Part model, mm, in its own coordinate system. A direction names the side the tool comes from. Coordinates: 2 decimals unless noted, no trailing zeros. Write each loop counter-clockwise with the first axis right and the second up, starting at its lowest first coordinate (ties: lowest second). Pieces come first, ordered by that corner, then holes. Notation, with made-up numbers: (18.25, 54) -> (70.25, 54) arc R19 ccw to (70.25, 88) -> close; hole circle Ø8 at (-18.5, 40.25). An arc over 180 degrees is marked (long way). Write item = value, one per line.
from build123d import *

# Parameters (mm, degrees)
SKETCH_1_R               = 38
SKETCH_1_R_2             = 36
EXTRUDE_1_DEPTH          = 34
EXTRUDE_START            = -2
SKETCH_2_R               = 40
SKETCH_2_R_2             = 38
EXTRUDE_2_DEPTH          = 2
EXTRUDE_START_2          = -34
SKETCH_2_2_R             = 40
SKETCH_2_2_R_2           = 38
EXTRUDE_3_DEPTH          = 2
SKETCH_3_R               = 36
SKETCH_3_R_2             = 34
EXTRUDE_4_DEPTH          = 40
SKETCH_4_R               = 34
EXTRUDE_5_DEPTH          = 2
CUT_EXTRUDE_1_DEPTH      = 94.145048178
CUT_EXTRUDE_1_DEPTH_BACK = 94.145048178
SKETCH_5_R               = 5
EXTRUDE_START_3          = -30
SKETCH_6_R               = 34
EXTRUDE_6_DEPTH          = 2
EXTRUDE_7_DEPTH          = 10
SKETCH_8_R               = 36
SKETCH_8_R_2             = 34
EXTRUDE_9_DEPTH          = 34


with BuildPart() as part:
    # Sketch 1 → Extrude 1 (new body)
    with BuildSketch(Plane.XY):
        Circle(SKETCH_1_R)
        Circle(SKETCH_1_R_2, mode=Mode.SUBTRACT)
    extrude(amount=EXTRUDE_1_DEPTH)

    # Sketch 2 → Extrude 2 (add)
    with BuildSketch(Plane.XY.offset(34).offset(EXTRUDE_START)):
        Circle(SKETCH_2_R)
        Circle(SKETCH_2_R_2, mode=Mode.SUBTRACT)
    extrude(amount=EXTRUDE_2_DEPTH)

    # Sketch 2_2 → Extrude 3 (add)
    with BuildSketch(Plane.XY.offset(34).offset(EXTRUDE_START_2)):
        Circle(SKETCH_2_2_R)
        Circle(SKETCH_2_2_R_2, mode=Mode.SUBTRACT)
    extrude(amount=EXTRUDE_3_DEPTH)



with BuildPart() as body_2:
    # Sketch 3 → Extrude 4 (new body)
    with BuildSketch(Plane(origin=(0, 0, 0), x_dir=(-1, 0, 0), z_dir=(0, 0, -1))):
        with Locations(Location((0, 0, 0), (0, 0, 180))):
            Circle(SKETCH_3_R)
        Circle(SKETCH_3_R_2, mode=Mode.SUBTRACT)
    extrude(amount=EXTRUDE_4_DEPTH)

    # Sketch 4 → Extrude 5 (add)
    with BuildSketch(Plane(origin=(0, 0, -40), x_dir=(-1, 0, 0), z_dir=(0, 0, -1))):
        Circle(SKETCH_4_R)
    extrude(amount=-EXTRUDE_5_DEPTH)

    # Sketch 5 → Cut-Extrude 1 (cut, two sides: drawn at the far end of the back side and taken through both)
    with BuildSketch(Plane(origin=(0, 0, -40), x_dir=(-1, 0, 0), z_dir=(0, 0, -1)).offset(-CUT_EXTRUDE_1_DEPTH_BACK)):
        Circle(SKETCH_5_R)
    extrude(amount=CUT_EXTRUDE_1_DEPTH + CUT_EXTRUDE_1_DEPTH_BACK, mode=Mode.SUBTRACT)

    # Sketch 6 → Extrude 6 (add)
    with BuildSketch(Plane.XY.offset(EXTRUDE_START_3)):
        Circle(SKETCH_6_R)
    extrude(amount=EXTRUDE_6_DEPTH)

    # Sketch 7 → Extrude 7 (add)
    with BuildSketch(Plane.XY.offset(-28)):
        Polygon((0, 7), (12, 7), (12, -7), (-12, -7), (-12, 7), align=None)
        Polygon((0, 5), (10, 5), (10, -5), (-10, -5), (-10, 5), align=None, mode=Mode.SUBTRACT)
    extrude(amount=EXTRUDE_7_DEPTH)


with BuildPart() as part_1:
    add(part.part)

    add(body_2.part)  # Extrude 9 merges body 2
    # Sketch 8 → Extrude 9 (add, through all)
    with BuildSketch(Plane.XY):
        Circle(SKETCH_8_R)
        Circle(SKETCH_8_R_2, mode=Mode.SUBTRACT)
    extrude(amount=EXTRUDE_9_DEPTH)


solid = part_1.part
Q1. Saw through at B-B on x = -26. Give the cut face in (y, z), and give its area (3 significant figures).
Model answer:
outline = (-30.4, 0) -> (-24.9, 0) -> (-24.9, -40) -> (24.9, -40) -> (24.9, 0) -> (30.4, 0) -> (30.4, 2) -> (27.71, 2) -> (27.71, 32) -> (30.4, 32) -> (30.4, 34) -> (21.91, 34) -> (21.91, -28) -> (-21.91, -28) -> (-21.91, 34) -> (-30.4, 34) -> (-30.4, 32) -> (-27.71, 32) -> (-27.71, 2) -> (-30.4, 2) -> close; hole (-21.91, -38) -> (21.91, -38) -> (21.91, -30) -> (-21.91, -30) -> close
area = 831 mm²
Q2. Pin check, flat tips, straight feed: pin 1 (5 mm diameter, centred on x = 4, z = -21.5, fed in from +Y); pin 2 (12 mm diameter, centred on y = 4, z = -24, fed in from -X); pin 3 (6 mm diameter, centred on x = 0, y = 0, fed in from +Z). Stop position of each tip, or through.
Model answer:
pin_1 = 35.97
pin_2 = -36
pin_3 = -28
Q3. Which spindle directions (+Z, -Z, +X, -X, +Y, -Y) get a long thin tool onto all of the face, cutting with end or side? Do faces 4 (the face through (-26.533, -24.331, -19.72)), 5 (the face through (35.4, -14.6, 2)), 6 (the face through (10, 0, -23)). Say none if no direction does.
Model answer:
face_4 = -Z
face_5 = none
face_6 = +Z
Q4. Mould opens along Y. For faces 1 (the face through (-33, 15, 0)), 2 (the face through (12, 0, -23)), 3 (the face through (-8.67, -39.05, 32.99)) say: released by +Y, released by -Y, zero draft, split by the parting line, or undercut.
Model answer:
face_1 = zero draft
face_2 = undercut
face_3 = split by the parting line
Q5. Saw through at C-C on z = 15. Give the cut face in (x, y), and give its area (3 significant figures).
Model answer:
outline = circle Ø76 at (0, 0); hole circle Ø68 at (0, 0)
area = 905 mm²
Q6. Probe line 1 (Y direction, x = 0, z = -18.5); line 2 (Z direction, x = -17.5, y = -6); line 3 (Y direction, x = 0, z = -6). List the from-to ranges inside material, lowest first. Write a range as from..to.
Model answer:
line_1 = -36..-34, -7..-5, 5..7, 34..36
line_2 = -40..-38, -30..-28
line_3 = -36..-34, 34..36
Q7. Saw through at A-A on y = 21. Give the cut face in (x, z), and give its area (3 significant figures).
Model answer:
outline = (-34.04, 0) -> (-29.24, 0) -> (-29.24, -40) -> (29.24, -40) -> (29.24, 0) -> (34.04, 0) -> (34.04, 2) -> (31.67, 2) -> (31.67, 32) -> (34.04, 32) -> (34.04, 34) -> (26.74, 34) -> (26.74, -28) -> (-26.74, -28) -> (-26.74, 34) -> (-34.04, 34) -> (-34.04, 32) -> (-31.67, 32) -> (-31.67, 2) -> (-34.04, 2) -> close; hole (-26.74, -38) -> (26.74, -38) -> (26.74, -30) -> (-26.74, -30) -> close
area = 768 mm²
